from build123d import *

# Parameters (mm, degrees)
SCHIZZO1_W                   = 20
SCHIZZO1_H                   = 45
ESTRUSIONE_ESTRUSIONE1_DEPTH = 33
SCHIZZO2_R                   = 7.5
TAGLIO_ESTRUSIONE1_DEPTH     = 60.279001341
FORO_4_0_4_1_D               = 4
FORO_4_0_4_1_DEPTH           = 10
FORO_4_0_4_1_TIP             = 1.201721238
SMUSSO1_SIZE                 = 3
SCHIZZO7_W                   = 11.145993212
SCHIZZO7_H                   = 24
TAGLIO_ESTRUSIONE4_DEPTH     = 26


with BuildPart() as part:
    # Schizzo1 → Estrusione-Estrusione1 (new body)
    with BuildSketch(Plane.XY):
        with Locations((10, 22.5)):
            Rectangle(SCHIZZO1_W, SCHIZZO1_H)
    extrude(amount=-ESTRUSIONE_ESTRUSIONE1_DEPTH)

    # Schizzo2 → Taglio-Estrusione1 (cut, through all)
    with BuildSketch(Plane.XZ):
        with Locations(Location((10, -11.9, 0), (0, 0, 270))):
            Circle(SCHIZZO2_R)
    extrude(amount=-TAGLIO_ESTRUSIONE1_DEPTH, mode=Mode.SUBTRACT)

    # Foro _4.0 _4_-1
    with Locations(Plane(origin=(10, 6, -33), x_dir=(-1, 0, 0), z_dir=(0, 0, -1))):
        with Locations((0, 0), (0, 33)):
            Hole(FORO_4_0_4_1_D / 2, depth=FORO_4_0_4_1_DEPTH)
            with Locations((0, 0, -(FORO_4_0_4_1_DEPTH + FORO_4_0_4_1_TIP / 2))):  # 118° drill point
                Cone(0, FORO_4_0_4_1_D / 2, FORO_4_0_4_1_TIP, mode=Mode.SUBTRACT)

    # Smusso1
    smusso1_edges = [part.edges().sort_by_distance(p)[0] for p in [
        (20, 22.5, 0),
        (0, 22.5, 0),
    ]]
    chamfer(smusso1_edges, length=SMUSSO1_SIZE)

    # Schizzo7 → Taglio-Estrusione4 (cut)
    with BuildSketch(Plane.ZY):
        with Locations((-27.427003394, 22.5)):
            Rectangle(SCHIZZO7_W, SCHIZZO7_H)
    extrude(amount=-TAGLIO_ESTRUSIONE4_DEPTH, mode=Mode.SUBTRACT)


solid = part.part
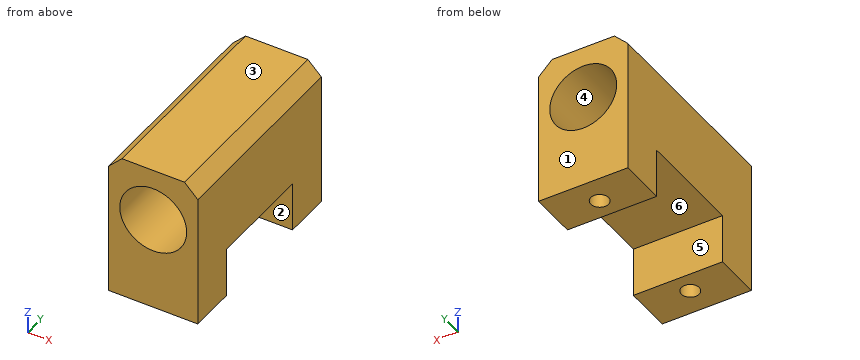
Input: part model. Units: mm. Frame: model coordinates. Face numbers are marked on the shaded views. A direction names the side the tool comes from. Round coordinates to 2 decimals unless told otherwise and drop trailing zeros. Write each loop counter-clockwise with the first axis right and the second up, starting at its lowest first coordinate (ties: lowest second). Pieces come first, ordered by that corner, then holes.
1) Ray query, L1, parallel to Y at x = 10, z = -25.25; L2, parallel to Z at x = 10.25, y = 28; L3, parallel to X at y = 39, z = -31. Return the intervals inside material, ascending.
2) Reachability of the marked faces 1 and 2 from +Z, -Z, +X, -X, +Y, -Y: full face, straight path, thin tool, end or side. Return the list, or none.
3) Cut plane B-B (x = 4.5). Return the cut outline in (y, z), then the cut area to 3 significant figures.
4) Cut plane C-C (z = -11.9). Return the cut outline in (x, y), then the cut area to 3 significant figures.
5) Contact query for flat-ended pins moving along their axis: P1, Ø6, axis at x = 11.5, y = 23.5, coming from the -Z side; P2, Ø6.5, axis at x = 10, y = 6, coming from the -Z side; P3, Ø6, axis at x = 10.5, z = -7.5, coming from the +Y side. Output: stop coordinate, or through.
6) Draft query along Z for the marked faces 3, 4, 5 and 6. Return one class per face: pulls with the +Z half, pulls with the -Z half, needs draft (parallel to the pull), parting line crosses it, or undercut.
7) Cut plane D-D (y = 13). Return the cut outline in (x, z), then the cut area to 3 significant figures.
8) Cut plane A-A (z = -26). Return the cut outline in (x, y).
Geometry says:
1. L1: y = 0 to 4, 8 to 10.5, 34.5 to 37, 41 to 45
1. L2: z = -21.85 to -19.4, -4.4 to 0
1. L3: x = 0 to 8, 12 to 20
2. face 1: +Z, -Z, +X, -X, +Y
2. face 2: -Z, +X, -X
3. outline: (0, -33) - (10.5, -33) - (10.5, -21.85) - (34.5, -21.85) - (34.5, -33) - (45, -33) - (45, -17) - (0, -17) - close; (0, -6.8) - (45, -6.8) - (45, 0) - (0, 0) - close
3. area: 759 mm2
4. outline: (0, 0) - (2.5, 0) - (2.5, 45) - (0, 45) - close; (17.5, 0) - (20, 0) - (20, 45) - (17.5, 45) - close
4. area: 225 mm2
5. P1: stops at z = -21.85
5. P2: stops at z = -33
5. P3: passes through
6. face 3: pulls with the +Z half
6. face 4: undercut
6. face 5: needs draft
6. face 6: pulls with the -Z half
7. outline: (0, -21.85) - (20, -21.85) - (20, -3) - (17, 0) - (3, 0) - (0, -3) - close; hole circle Ø15 at (10, -11.9)
7. area: 251 mm2
8. outline: (0, 0) - (20, 0) - (20, 10.5) - (0, 10.5) - close; (0, 34.5) - (20, 34.5) - (20, 45) - (0, 45) - close; hole circle Ø4 at (10, 6); hole circle Ø4 at (10, 39)
